from build123d import *

# Parameters (mm, degrees)
EXTRUDE_1_DEPTH     = 10
SKETCH_2_R          = 17.9
SKETCH_2_R_2        = 25.15
CUT_EXTRUDE_1_DEPTH = 178.623196683
SKETCH_4_R          = 34.15
CUT_EXTRUDE_2_DEPTH = 1.8
SKETCH_5_R          = 32.65
CUT_EXTRUDE_3_DEPTH = 7.1
EXTRUDE_START       = 9.8
SKETCH_6_R          = 20.9
SKETCH_6_R_2        = 17.9
EXTRUDE_2_DEPTH     = 9.8
EXTRUDE_START_2     = -10
EXTRUDE_3_DEPTH     = 10
CUT_EXTRUDE_4_DEPTH = 192.421106464
SKETCH_11_R         = 3.5
CUT_EXTRUDE_5_DEPTH = 191.656759649
CUT_EXTRUDE_6_DEPTH = 191.656759649


with BuildPart() as part:
    # 草图1 → 凸台-拉伸1 (new body)
    with BuildSketch(Plane(origin=(0, 0, 0), x_dir=(1, 0, 0), z_dir=(0, 1, 0))):
        with BuildLine():
            Line((63.686733312, -87), (44.09081537, 9))
            ThreePointArc((44.09081537, 9), (0, 45), (-44.09081537, 9))
            Line((-44.09081537, 9), (-63.686733312, -87))
            ThreePointArc((-63.686733312, -87), (0, -165), (63.686733312, -87))
        make_face()
    extrude(amount=EXTRUDE_1_DEPTH)

    # 草图2 → 切除-拉伸1 (cut, through all)
    with BuildSketch(Plane(origin=(0, 10, 0), x_dir=(1, 0, 0), z_dir=(0, 1, 0))):
        with Locations(Location((0, 0, 0), (0, 0, 270))):
            Circle(SKETCH_2_R)
        with Locations(Location((0, -100, 0), (0, 0, 270))):
            Circle(SKETCH_2_R_2)
    extrude(amount=-CUT_EXTRUDE_1_DEPTH, mode=Mode.SUBTRACT)

    # 草图4 → 切除-拉伸2 (cut)
    with BuildSketch(Plane(origin=(0, 10, 0), x_dir=(1, 0, 0), z_dir=(0, 1, 0))):
        with Locations(Location((0, -100, 0), (0, 0, 270))):
            Circle(SKETCH_4_R)
    extrude(amount=-CUT_EXTRUDE_2_DEPTH, mode=Mode.SUBTRACT)

    # 草图5 → 切除-拉伸3 (cut)
    with BuildSketch(Plane(origin=(0, 8.2, 0), x_dir=(1, 0, 0), z_dir=(0, 1, 0))):
        with Locations(Location((0, -100, 0), (0, 0, 270))):
            Circle(SKETCH_5_R)
    extrude(amount=-CUT_EXTRUDE_3_DEPTH, mode=Mode.SUBTRACT)

    # 草图6 → 凸台-拉伸2 (add)
    with BuildSketch(Plane(origin=(0, 10, 0), x_dir=(1, 0, 0), z_dir=(0, 1, 0)).offset(EXTRUDE_START)):
        with Locations(Location((0, 0, 0), (0, 0, 270))):
            Circle(SKETCH_6_R)
        with Locations(Location((0, 0, 0), (0, 0, 270))):
            Circle(SKETCH_6_R_2, mode=Mode.SUBTRACT)
    extrude(amount=-EXTRUDE_2_DEPTH)

    # 草图7 → 凸台-拉伸3 (add)
    with BuildSketch(Plane.XZ.offset(EXTRUDE_START_2)):
        with BuildLine():
            Line((-44.09081537, -9), (-45, -4.54592315))
            Line((-45, -4.54592315), (-45, -40))
            Line((-45, -40), (-20.615528128, -40))
            ThreePointArc((-20.615528128, -40), (-35.874471734, -27.166565439), (-44.09081537, -9))
        make_face()
        with BuildLine():
            ThreePointArc((56.203418539, 50.33939444), (0, 175), (-56.203418539, 50.33939444))
            Line((-56.203418539, 50.33939444), (-63.686733312, 87))
            ThreePointArc((-63.686733312, 87), (0, 165), (63.686733312, 87))
            Line((63.686733312, 87), (56.203418539, 50.33939444))
        make_face()
        with BuildLine():
            Line((45, -40), (45, -4.54592315))
            Line((45, -4.54592315), (44.09081537, -9))
            ThreePointArc((44.09081537, -9), (35.874471734, -27.166565439), (20.615528128, -40))
            Line((20.615528128, -40), (45, -40))
        make_face()
    extrude(amount=EXTRUDE_3_DEPTH)

    # 草图8 → 切除-拉伸4 (cut, through all)
    with BuildSketch(Plane.XZ):
        with BuildLine():
            Line((-45, -4.54592315), (-45, 40))
            ThreePointArc((-45, 40), (-50.865103463, 44.884292169), (-56.203418539, 50.33939444))
            Line((-56.203418539, 50.33939444), (-45, -4.54592315))
        make_face()
        with BuildLine():
            ThreePointArc((56.203418539, 50.33939444), (50.865103463, 44.884292169), (45, 40))
            Line((45, 40), (45, -4.54592315))
            Line((45, -4.54592315), (56.203418539, 50.33939444))
        make_face()
        with BuildLine():
            Line((20.615528128, -40), (-20.615528128, -40))
            ThreePointArc((-20.615528128, -40), (0, -45), (20.615528128, -40))
        make_face()
    extrude(amount=-CUT_EXTRUDE_4_DEPTH, mode=Mode.SUBTRACT)

    # 草图11 → 切除-拉伸5 (cut, through all)
    with BuildSketch(Plane(origin=(0, 10, 0), x_dir=(1, 0, 0), z_dir=(0, 1, 0))):
        with Locations(Location((0, -167.7, 0), (0, 0, 270))):
            Circle(SKETCH_11_R)
        with Locations(Location((47.871129086, -147.871129086, 0), (0, 0, 270))):
            Circle(SKETCH_11_R)
        with Locations(Location((-47.871129086, -147.871129086, 0), (0, 0, 270))):
            Circle(SKETCH_11_R)
        with Locations(Location((-67.7, -100, 0), (0, 0, 270))):
            Circle(SKETCH_11_R)
        with Locations(Location((-47.871129086, -52.128870914, 0), (0, 0, 270))):
            Circle(SKETCH_11_R)
        with Locations(Location((67.7, -100, 0), (0, 0, 270))):
            Circle(SKETCH_11_R)
        with Locations(Location((47.871129086, -52.128870914, 0), (0, 0, 270))):
            Circle(SKETCH_11_R)
    extrude(amount=-CUT_EXTRUDE_5_DEPTH, mode=Mode.SUBTRACT)

    # 草图12 → 切除-拉伸6 (cut, through all)
    with BuildSketch(Plane(origin=(0, 10, 0), x_dir=(1, 0, 0), z_dir=(0, 1, 0))):
        with BuildLine():
            ThreePointArc((-45, -40), (-40.12511839, -36.636170616), (-35, -33.667504193))
            Line((-35, -33.667504193), (-35, 40))
            Line((-35, 40), (-45, 40))
            Line((-45, 40), (-45, -40))
        make_face()
        with BuildLine():
            Line((35, 40), (35, -33.667504193))
            ThreePointArc((35, -33.667504193), (40.12511839, -36.636170616), (45, -40))
            Line((45, -40), (45, 40))
            Line((45, 40), (35, 40))
        make_face()
    extrude(amount=-CUT_EXTRUDE_6_DEPTH, mode=Mode.SUBTRACT)


solid = part.part
Can you work these out from the model? Positions are in its coordinate system, mm. A direction names the side the tool comes from. Coordinates: 2 decimals unless noted, no trailing zeros. Write each loop counter-clockwise with the first axis right and the second up, starting at its lowest first coordinate (ties: lowest second). Pieces come first, ordered by that corner, then holes. Notation, with made-up numbers: (37.25, -6) - (69.25, -6) arc R18 cw to (69.25, 2) - close; hole circle Ø11 at (12, 57). An arc over 180 degrees is marked (long way). Return JSON: item names as keys, results as strings. Group by question number.
Item 1: Please list where these lines run through material, in increasing order: probe 1 along X at (y, z) = (8.6, 100); probe 2 along X at (y, z) = (6, 148.5); probe 3 along Y at (x, z) = (49, 155).
Item 2: We'd pull the mould along X, two halves only. Please class faces 4 (the face through (-46.82, 5.07, 55.467)), 5 (the face through (35, 5, -4)), 6 (the face through (6.278, 14.969, 19.935)): pulls with the +X half, pulls with the -X half, needs draft (parallel to the pull), parting line crosses it, or undercut.
Item 3: If we section it at B-B (x = 0): Write out the boundary of the cut face in (y, z), then the cut area to 3 significant figures.
Item 4: I'm going to push flat-ended pins straight in: pin 1 Ø21.5 at (x, z) = (0, 0) entering from +Y; pin 2 Ø8 at (y, z) = (3, -8.5) entering from -X; pin 3 Ø11 at (x, z) = (47.87, 52.13) entering from +Y; pin 4 Ø1.5 at (x, z) = (7, 74) entering from +Y. Where does each tip first touch, or does it pass through?
Item 5: If we section it at A-A (z = 100): Write out the boundary of the cut face in (x, y).
Item 6: If we section it at C-C (z = 0): Write out the boundary of the cut face in (x, y).
Item 7: If we section it at D-D (x = -67.7): Write out the boundary of the cut face in (y, z).
Item 8: Which directions (+Z, -Z, +X, -X, +Y, -Y) give clear straight access to the entire face, cutting with the end or side of a thin tool? Please do faces 1 (the face through (66.359, 5.07, 103.233)), 2 (the face through (-35, 5, -3)), 3 (the face through (-19, 1.1, 117)).
Return value:
{
 "1": {"probe 1": "x = -75 to -71.2, -64.2 to -34.15, 34.15 to 64.2, 71.2 to 75", "probe 2": "x = -57.21 to -51.31, -44.43 to 44.43, 51.31 to 57.21", "probe 3": "y = 0 to 10"},
 "2": {"face 4": "undercut", "face 5": "pulls with the +X half", "face 6": "parting line crosses it"},
 "3": {"outline": "(0, -40) - (10, -40) - (10, -20.9) - (19.8, -20.9) - (19.8, -17.9) - (0, -17.9) - close; (0, 17.9) - (19.8, 17.9) - (19.8, 20.9) - (10, 20.9) - (10, 65.85) - (8.2, 65.85) - (8.2, 67.35) - (1.1, 67.35) - (1.1, 74.85) - (0, 74.85) - close; (0, 125.15) - (1.1, 125.15) - (1.1, 132.65) - (8.2, 132.65) - (8.2, 134.15) - (10, 134.15) - (10, 164.2) - (0, 164.2) - close; (0, 171.2) - (10, 171.2) - (10, 175) - (0, 175) - close", "area": "1,140 mm^2"},
 "4": {"pin 1": "passes through", "pin 2": "stops at x = -35", "pin 3": "stops at y = 10", "pin 4": "stops at y = 1.1"},
 "5": {"outline": "(-75, 0) - (-71.2, 0) - (-71.2, 10) - (-75, 10) - close; (-64.2, 0) - (-25.15, 0) - (-25.15, 1.1) - (-32.65, 1.1) - (-32.65, 8.2) - (-34.15, 8.2) - (-34.15, 10) - (-64.2, 10) - close; (25.15, 0) - (64.2, 0) - (64.2, 10) - (34.15, 10) - (34.15, 8.2) - (32.65, 8.2) - (32.65, 1.1) - (25.15, 1.1) - close; (71.2, 0) - (75, 0) - (75, 10) - (71.2, 10) - close"},
 "6": {"outline": "(-35, 0) - (-17.9, 0) - (-17.9, 19.8) - (-20.9, 19.8) - (-20.9, 10) - (-35, 10) - close; (17.9, 0) - (35, 0) - (35, 10) - (20.9, 10) - (20.9, 19.8) - (17.9, 19.8) - close"},
 "7": {"outline": "(0, 67.72) - (10, 67.72) - (10, 96.5) - (0, 96.5) - close; (0, 103.5) - (10, 103.5) - (10, 132.28) - (0, 132.28) - close"},
 "8": {"face 1": "+Y, -Y", "face 2": "-Z, -X, +Y, -Y", "face 3": "+Y"}
}
